from build123d import *

# Parameters (mm, degrees)
BOSS_EXTRU_1_DEPTH                        = 10
TROU_POUR_TARAUDAGE_POUR_TROU_TARAUD_M3_D = 2.5


with BuildPart() as part:
    # Esquisse1 → Boss.-Extru.1 (new body)
    with BuildSketch(Plane.XY):
        Polygon((0, 3.464101615), (-3, 1.732050808), (-3, -1.732050808), (0, -3.464101615), (3, -1.732050808), (3, 1.732050808), align=None)
    extrude(amount=BOSS_EXTRU_1_DEPTH)

    # Esquisse2 → Enlèvement de matière-Révolution1 (revolve, cut)
    with BuildSketch(Plane(origin=(0, 0, 0), x_dir=(0, 0, -1), z_dir=(1, 0, 0))):
        Polygon((-10, 2.964101615), (-9.5, 3.464101615), (-9.5, 7.964101615), (-14.5, 7.964101615), (-14.5, 2.964101615), align=None)
        Polygon((0, 2.964101615), (4.5, 2.964101615), (4.5, 7.964101615), (-0.5, 7.964101615), (-0.5, 3.464101615), align=None)
    revolve(axis=Axis((0, 0, 1000), (0, 0, -1)), mode=Mode.SUBTRACT)

    # Trou pour taraudage pour trou taraudé M31 (through all)
    with Locations(Plane(origin=(0, 0, 0), x_dir=(-1, 0, 0), z_dir=(0, 0, -1))):
        with Locations((0, 0)):
            Hole(TROU_POUR_TARAUDAGE_POUR_TROU_TARAUD_M3_D / 2)


solid = part.part
Design review of the part built by this model. Coordinates are the model's own, in mm. Coordinates: 2 decimals unless noted, no trailing zeros. Order: outer loops, then holes, each group sorted by start corner. A loop starts at its lowest first (then second) coordinate and runs counter-clockwise, first axis right, second up. Notation, with made-up numbers: (-32, 40.5) -> (-16, 40.5) arc R18 ccw to (-16, 71.5) -> close; hole circle Ø9 at (54.25, 49). An arc over 180 degrees is marked (long way). One line per item, written item: value.
1) Draft analysis for pull direction Y (two halves, no side actions). For faces 1 (the face through (-0.27, -1.22, 5.07)), 2 (the face through (1, -1, 10)), 3 (the face through (-1.5, 2.6, 4.9)), state which applies: +Y half, -Y half, draft (parallel to the pull), parting line (faces both ways), or undercut.
Output values:
face 1: undercut
face 2: draft
face 3: +Y half
2) We need section A-A, the plane z = 5.75. Give the boundary of the cut face in (x, y).
Output values:
outline: (-3, -1.73) -> (0, -3.46) -> (3, -1.73) -> (3, 1.73) -> (0, 3.46) -> (-3, 1.73) -> close; hole circle Ø2.5 at (0, 0)
3) To check wall thickness, follow probe 1 along X at (y, z) = (-1, 2.25); probe 2 along Y at (x, z) = (0.4, 3.25); probe 3 along Y at (x, z) = (-0.3, 7). State the ranges of each line that lie inside material, in increasing order. Write a range as [from, to].
Output values:
probe 1: x = [-3, -0.75], [0.75, 3]
probe 2: y = [-3.23, -1.18], [1.18, 3.23]
probe 3: y = [-3.29, -1.21], [1.21, 3.29]
